Job drawing, mm, ordinate dimensions from the low corner. One solid piece. A direction names the side the tool comes from. Coordinates: 2 decimals unless noted, no trailing zeros. Loops run counter-clockwise (first coordinate to the right, second up) from the corner with the lowest first, then second, coordinate; pieces in that order, holes last. Notation, with made-up numbers: M 54,35 L 102,35 A31 cw 102,66 Z; hole C -39.5,53 d8. An arc over 180 degrees is marked long. Answer as a JSON object with one key per item and string values. Group by question number.
1. Saw through at D-D on z = 216. Write the cut outline in (x, y), then the cut area to 3 significant figures.
2. Drop flat-ended pins along their axis: pin 1 Ø8 at (x, y) = (181, 22.5) entering from +Z; pin 2 Ø5 at (x, y) = (38.5, 7) entering from -Z; pin 3 Ø4 at (x, y) = (124, 7) entering from -Z. Give the stop position or say it passes through.
3. Saw through at A-A on z = 152.4. Write the cut outline in (x, y).
4. Saw through at B-B on x = 152.4. Write the cut outline in (y, z).
5. Mould opens along Z. For the marked faces 3, 4 and 5 say: released by +Z, released by -Z, zero draft, split by the parting line, or undercut.
6. Drill centre lines: L1, parallel to Z at x = 148.5, y = 2; L2, parallel to Z at x = 42, y = 30.5; L3, parallel to Y at x = 75, z = 283.5. Where is each one in solid material? Low to high.
7. 3-axis set-ups, long thin cutter, end or side, ignore diameter. For the marked faces 1 and 2: which of +Z, -Z, +X, -X, +Y, -Y reach the whole face in a straight line?
8. Saw through at C-C on y = 15.5. Write the cut outline in (x, z), then the cut area to 3 significant figures.
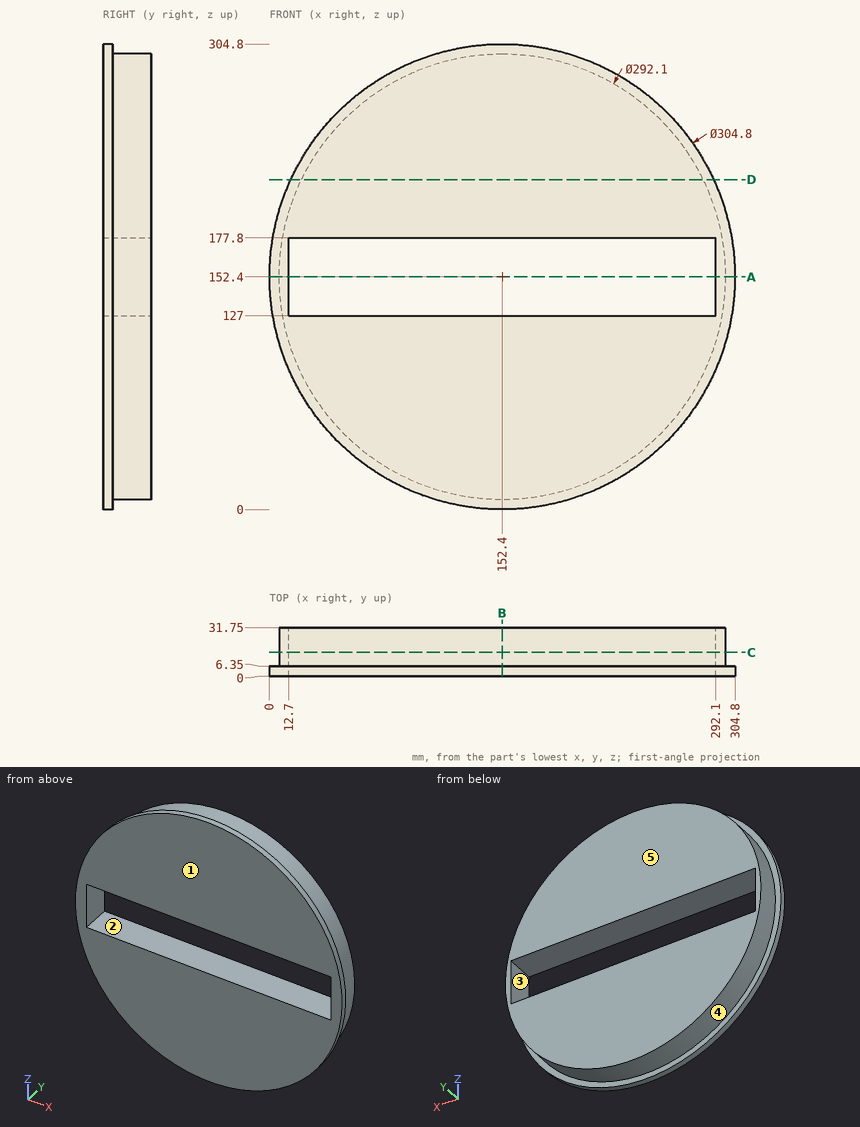
Outcome:
{
 "1": {"outline": "M 13.91,0 L 290.89,0 L 290.89,6.35 L 283.87,6.35 L 283.87,31.75 L 20.93,31.75 L 20.93,6.35 L 13.91,6.35 Z", "area": "8,440 mm²"},
 "2": {"pin 1": "stops at z = 296.36", "pin 2": "stops at z = 48.49", "pin 3": "stops at z = 2.32"},
 "3": {"outline": "M 0,0 L 12.7,0 L 12.7,31.75 L 6.35,31.75 L 6.35,6.35 L 0,6.35 Z; M 292.1,0 L 304.8,0 L 304.8,6.35 L 298.45,6.35 L 298.45,31.75 L 292.1,31.75 Z"},
 "4": {"outline": "M 0,0 L 6.35,0 L 6.35,6.35 L 31.75,6.35 L 31.75,127 L 0,127 Z; M 0,177.8 L 31.75,177.8 L 31.75,298.45 L 6.35,298.45 L 6.35,304.8 L 0,304.8 Z"},
 "5": {"face 3": "undercut", "face 4": "split by the parting line", "face 5": "zero draft"},
 "6": {"L1": "z = 0.05 to 127, 177.8 to 304.75", "L2": "z = 56.78 to 127, 177.8 to 248.02", "L3": "y = 0 to 6.35"},
 "7": {"face 1": "+Z, -Z, +X, -X, -Y", "face 2": "+Y, -Y"},
 "8": {"outline": "C 152.4,152.4 d292.1; hole M 12.7,127 L 292.1,127 L 292.1,177.8 L 12.7,177.8 Z", "area": "52,800 mm²"}
}
